Verification items for the finished model (mm, model axes). Face numbers are marked on the shaded views. A direction names the side the tool comes from. Round coordinates to 2 decimals unless told otherwise and drop trailing zeros. Write each loop counter-clockwise with the first axis right and the second up, starting at its lowest first coordinate (ties: lowest second). Pieces come first, ordered by that corner, then holes. Notation, with made-up numbers: M 69,56.5 L 83,56.5 A31 cw 83,80.5 Z; hole C -32,-10.5 d4. An arc over 180 degrees is marked long. One line per question, with ' | ' between items.
from build123d import *

# Parameters (mm, degrees)
SKETCH1_R           = 1.5
BOSS_EXTRUDE1_DEPTH = 6


with BuildPart() as part:
    # Sketch1 → Boss-Extrude1 (new body)
    # profile 1 of 2: a face of its own
    with BuildSketch(Plane.XY):
        with BuildLine():
            ThreePointArc((4, 0), (4.32733046, -4.052535377), (5.300835088, -8))
            Line((5.300835088, -8), (13.805264562, -8))
            ThreePointArc((13.805264562, -8), (21.532676707, -2.070531706), (17.805227526, 6.928224613))
            Line((17.805227526, 6.928224613), (12.501235753, 9.990447886))
            ThreePointArc((12.501235753, 9.990447886), (4.438362285, 11.989459523), (-3.451860404, 9.391313647))
            ThreePointArc((-3.451860404, 9.391313647), (-9.98812759, -3.562916176), (-2.498625359, -15.990394414))
            Line((-2.498625359, -15.990394414), (-1.533326535, -16.54770307))
            ThreePointArc((-1.533326535, -16.54770307), (-1.322910636, -14.159598792), (-1.82950584, -11.816379171))
            ThreePointArc((-1.82950584, -11.816379171), (-3.45287502, -6.00703466), (-4, 0))
            ThreePointArc((-4, 0), (0, 4), (4, 0))
        make_face()
    # profile 2 of 2: a face of its own
    with BuildSketch(Plane.XY):
        with BuildLine():
            ThreePointArc((-2.498625359, -15.990394414), (-9.98812759, -3.562916176), (-3.451860404, 9.391313647))
            ThreePointArc((-3.451860404, 9.391313647), (-5.601136209, 8.355737746), (-7.960215392, 8))
            Line((-7.960215392, 8), (-62, 8))
            ThreePointArc((-62, 8), (-65.911631869, 6.978476633), (-68.824307899, 4.17478403))
            ThreePointArc((-68.824307899, 4.17478403), (-68.429059963, -4.761007035), (-59.997026703, -7.745198382))
            ThreePointArc((-59.997026703, -7.745198382), (-32.671781582, -19.77866562), (-38.011446212, -49.154869194))
            ThreePointArc((-38.011446212, -49.154869194), (-40.527279582, -53.683744804), (-39.740705478, -58.804431575))
            ThreePointArc((-39.740705478, -58.804431575), (-32.818486758, -63.093194538), (-25.724521947, -59.094912029))
            Line((-25.724521947, -59.094912029), (-2.379078452, -18.659417769))
            ThreePointArc((-2.379078452, -18.659417769), (-1.880761637, -17.633774846), (-1.533326535, -16.54770307))
            Line((-1.533326535, -16.54770307), (-2.498625359, -15.990394414))
        make_face()
        with Locations((-32.652725178, -55.094912029)):
            Circle(SKETCH1_R, mode=Mode.SUBTRACT)
        with Locations((-62, 0)):
            Circle(SKETCH1_R, mode=Mode.SUBTRACT)
        with BuildLine():
            ThreePointArc((-49.5, -2.75), (-52.25, 0), (-49.5, 2.75))
            Line((-49.5, 2.75), (-42.5, 2.75))
            ThreePointArc((-42.5, 2.75), (-39.75, 0), (-42.5, -2.75))
            Line((-42.5, -2.75), (-49.5, -2.75))
        make_face(mode=Mode.SUBTRACT)
        with Locations((-30, 0)):
            Circle(SKETCH1_R, mode=Mode.SUBTRACT)
    extrude(amount=BOSS_EXTRUDE1_DEPTH)


solid = part.part
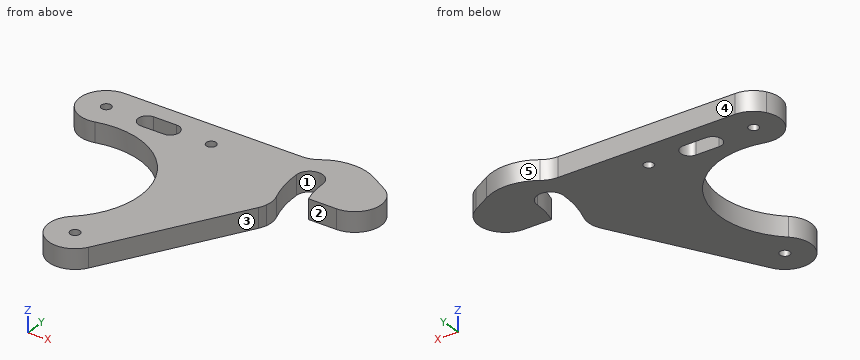
1. Section check B-B, the plane z = 3.6. Record the cut outline in (x, y).
Results:
outline: M -62,8 A8 ccw long -60,-7.75 A24.1 cw -38.01,-49.15 A8 ccw long -25.72,-59.09 L -2.38,-18.66 A8 ccw -1.83,-11.82 A33.25 cw -4,0 A4 cw 4,0 A25.25 ccw 5.3,-8 L 13.81,-8 A8 ccw 17.81,6.93 L 12.5,9.99 A15 ccw -3.45,9.39 A8 cw -7.96,8 Z; hole C -62,0 d3; hole M -49.5,-2.75 L -42.5,-2.75 A2.75 ccw -42.5,2.75 L -49.5,2.75 A2.75 ccw Z; hole C -32.65,-55.09 d3; hole C -30,0 d3
2. Section check A-A, the plane x = -45.5. Record the cut outline in (y, z), then the cut area to 3 significant figures.
Results:
outline: M -8.51,0 L -2.75,0 L -2.75,6 L -8.51,6 Z; M 2.75,0 L 8,0 L 8,6 L 2.75,6 Z | area: 66.1 mm2
3. Tool access check on the marked faces 4 and 5. Record the directions out of +Z, -Z, +X, -X, +Y, -Y that give a thin tool (end or side, any length) a straight path to the whole face; none if there is none.
Results:
face 4: +Z, -Z, -X, +Y | face 5: +Z, -Z, +Y
4. Mould release check, pull along X, two halves, no side actions. Record for the marked faces 1, 2 and 3: pulls with the +X half, pulls with the -X half, needs draft (parallel to the pull), parting line crosses it, or undercut.
Results:
face 1: undercut | face 2: needs draft | face 3: pulls with the +X half
5. Section check C-C, the plane y = -34.5. Record the cut outline in (x, z).
Results:
outline: M -30.1,0 L -11.52,0 L -11.52,6 L -30.1,6 Z
6. Thickness scan on line 1 (Y direction, x = -62, z = 2.65); line 2 (Y direction, x = -54, z = 1.2); line 3 (Y direction, x = -50, z = 3.35). Record the ranges inside material, lowest first.
Results:
line 1: y = -8 to -1.5, 1.5 to 8 | line 2: y = -6.98 to 8 | line 3: y = -7.31 to -2.7, 2.7 to 8
7. Section check D-D, the plane x = -56. Record the cut outline in (y, z), then the cut area to 3 significant figures.
Results:
outline: M -7.06,0 L 8,0 L 8,6 L -7.06,6 Z | area: 90.4 mm2
8. Go/stop test with flat-tipped pins: P1, Ø2.5, axis at x = -62, y = 0, coming from the -Z side; P2, Ø5, axis at x = -32.65, y = -55.09, coming from the +Z side; P3, Ø1, axis at x = -42, z = 1, coming from the -Y side; P4, Ø1, axis at y = -22.5, z = 3.5, coming from the +X side. Record where each tip stops, or that it passes through.
Results:
P1: passes through | P2: stops at z = 6 | P3: stops at y = -10.45 | P4: stops at x = -4.31
